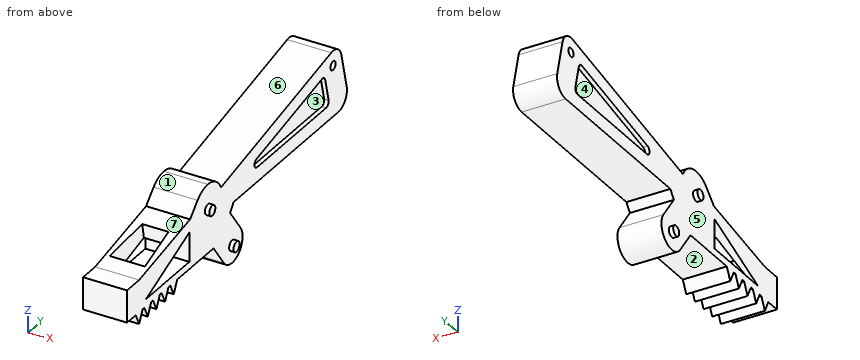
from build123d import *

# Parameters (mm, degrees)
BOSS_EXTRUDE1_DEPTH = 7.5
BOSS_EXTRUDE2_DEPTH = 15
LPATTERN1_COUNT     = 5
LPATTERN1_PITCH     = 5
CUT_EXTRUDE1_DEPTH  = 132.304814948
FILLET1_R           = 8.5
FILLET2_R           = 5
SKETCH4_R           = 1.5
CUT_EXTRUDE2_DEPTH  = 130.82329799
CUT_EXTRUDE3_REACH  = 131.114
SKETCH6_R           = 1.75
BOSS_EXTRUDE3_DEPTH = 1.5
SKETCH7_R           = 1.75
BOSS_EXTRUDE4_DEPTH = 1.5
CUT_EXTRUDE4_DEPTH  = 1.5


with BuildPart() as part:
    # Sketch1 → Boss-Extrude1 (new, symmetric)
    with BuildSketch(Plane(origin=(0, 0, 0), x_dir=(0, 0, -1), z_dir=(1, 0, 0))):
        with BuildLine():
            Line((1.125844004, 128.547240234), (-22.171185278, 122.781095368))
            Line((-22.171185278, 122.781095368), (-7.570249068, 54.320795472))
            Line((-7.570249068, 54.320795472), (-12.460270489, 53.277871457))
            Line((-12.460270489, 53.277871457), (-12.460270489, 43.277871457))
            Line((-12.460270489, 43.277871457), (-5.749067667, 36.443984461))
            Line((-5.749067667, 36.443984461), (0, 7))
            Line((0, 7), (0, 0))
            Line((0, 0), (11, 0))
            Line((11, 0), (11, 50))
            Line((11, 50), (19.022755483, 55.969538882))
            ThreePointArc((19.022755483, 55.969538882), (20.254685443, 64.364915501), (11.859308824, 65.596845461))
            Line((11.859308824, 65.596845461), (3.836553342, 59.627306579))
            Line((3.836553342, 59.627306579), (1.125844004, 61.629450689))
            Line((1.125844004, 61.629450689), (1.125844004, 128.547240234))
        make_face()
    extrude(amount=BOSS_EXTRUDE1_DEPTH, both=True)

    # Sketch2 → Boss-Extrude2 (add)
    with BuildSketch(Plane(origin=(7.5, 0, 0), x_dir=(0, 0, -1), z_dir=(1, 0, 0))):
        Polygon((11, 5), (15, 7), (11, 9), align=None)
    boss_extrude2 = extrude(amount=-BOSS_EXTRUDE2_DEPTH)

    # LPattern1: Boss-Extrude2 ×5
    with Locations(*[(0, i * LPATTERN1_PITCH, 0) for i in range(1, LPATTERN1_COUNT)]):
        add(boss_extrude2)

    # Sketch3 → Cut-Extrude1 (cut, through all)
    with BuildSketch(Plane(origin=(7.5, 0, 0), x_dir=(0, 0, -1), z_dir=(1, 0, 0))):
        Polygon((8.514249155, 11.015619925), (8.514249155, 36.015619925), (-1.485750845, 36.015619925), align=None)
    extrude(amount=-CUT_EXTRUDE1_DEPTH, mode=Mode.SUBTRACT)

    # Fillet1
    # the kernel refuses this fillet: 8.5 mm, written as the material it takes off along each edge
    with BuildSketch(Plane(origin=(-16.189504631, 43.277871457, 12.460270489), x_dir=(0, 1, 0), z_dir=(1, 0, 0))) as fillet1_piece_1:
        with BuildLine():
            CenterArc((FILLET1_R * 0.408917864968, -FILLET1_R), FILLET1_R, 90, 44.481059687)
            Line((-FILLET1_R * 0.29175558125, -FILLET1_R * 0.286517889667), (-FILLET1_R * 0.305769050174, -FILLET1_R * 0.27224824746))
            Line((-FILLET1_R * 0.305769050174, -FILLET1_R * 0.27224824746), (-FILLET1_R * 0.00817835729936, FILLET1_R * 0.02))
            Line((-FILLET1_R * 0.00817835729936, FILLET1_R * 0.02), (FILLET1_R * 0.408917864968, FILLET1_R * 0.02))
            Line((FILLET1_R * 0.408917864968, FILLET1_R * 0.02), (FILLET1_R * 0.408917864968, 0))
        make_face()
    extrude(amount=32.379009261, mode=Mode.SUBTRACT)
    with BuildSketch(Plane(origin=(-24.131006979, 53.277871457, 12.460270489), x_dir=(0, 0.20858480299843193, -0.9780042842227765), z_dir=(1, 0, 0))) as fillet1_piece_2:
        with BuildLine():
            CenterArc((6.92544629, -8.279049256), FILLET1_R, 103.092457682, 64.868111345)
            Line((-1.387590126, -6.506078431), (-1.553850854, -6.470619014))
            Line((-1.553850854, -6.470619014), (-0.166260728, 0.035459417))
            Line((-0.166260728, 0.035459417), (0, 0.17))
            ThreePointArc((0, 0.17), (2.5, 0.17), (4.961491074, 0.165580985))
            Line((4.961491074, 0.165580985), (5, 0))
        make_face()
    extrude(amount=48.262013958, mode=Mode.SUBTRACT)

    # Fillet2
    fillet2_edges = [part.edges().sort_by_distance(p)[0] for p in [
        (0, 122.781095368, 22.171185278),
        (0, 128.547240234, -1.125844004),
    ]]
    fillet(fillet2_edges, radius=FILLET2_R)

    # Sketch4 → Cut-Extrude2 (cut, through all)
    with BuildSketch(Plane(origin=(7.5, 0, 0), x_dir=(0, 0, -1), z_dir=(1, 0, 0))):
        with Locations((-16.271597688, 119.090404926)):
            Circle(SKETCH4_R)
    extrude(amount=-CUT_EXTRUDE2_DEPTH, mode=Mode.SUBTRACT)

    # Cut-Extrude3: up to this plane
    cut_extrude3_end = Plane(origin=(-7.5, 36.015619925, 1.485750845), z_dir=(0, -0.3713906763541038, 0.9284766908852593))
    # Sketch5 → Cut-Extrude3 (cut, up to the surface)
    with BuildSketch(Plane(origin=(0, 0.257069393, -1.316586904), x_dir=(1, 0, 0), z_dir=(0, -0.19163558890630344, 0.9814661487104557)), mode=Mode.PRIVATE) as cut_extrude3_sk1:
        Polygon((4.5, 29.370263041), (-4.5, 29.370263041), (-6, 12.858555839), (6, 12.858555839), align=None)
    cut_extrude3_tool1 = split(extrude(cut_extrude3_sk1.sketch, amount=-CUT_EXTRUDE3_REACH, mode=Mode.PRIVATE), bisect_by=cut_extrude3_end, keep=Keep.BOTH, mode=Mode.PRIVATE)
    add(cut_extrude3_tool1.solids().sort_by_distance((0, 20.594298, 2.654347))[0], mode=Mode.SUBTRACT)

    # Sketch6 → Boss-Extrude3 (add)
    with BuildSketch(Plane(origin=(7.5, 0, 0), x_dir=(0, 0, -1), z_dir=(1, 0, 0))):
        with Locations(Location((15.441032154, 60.783192172, 0), (0, 0, 180))):
            Circle(SKETCH6_R)
    boss_extrude3 = extrude(amount=BOSS_EXTRUDE3_DEPTH)

    # Sketch7 → Boss-Extrude4 (add)
    with BuildSketch(Plane(origin=(7.5, 0, 0), x_dir=(0, 0, -1), z_dir=(1, 0, 0))):
        with Locations(Location((-3.960270489, 46.753673309, 0), (0, 0, 180))):
            Circle(SKETCH7_R)
    boss_extrude4 = extrude(amount=BOSS_EXTRUDE4_DEPTH)

    # Sketch8 → Cut-Extrude4 (cut)
    with BuildSketch(Plane(origin=(7.5, 0, 0), x_dir=(0, 0, -1), z_dir=(1, 0, 0))):
        with BuildLine():
            Line((-14.925252721, 112.777715187), (-6.841162422, 74.873348079))
            ThreePointArc((-6.841162422, 74.873348079), (-5.216849988, 73.694496481), (-3.874155996, 75.186225283))
            Line((-3.874155996, 75.186225283), (-3.874155996, 115.091449891))
            ThreePointArc((-3.874155996, 115.091449891), (-4.449649663, 116.272673004), (-5.73454005, 116.547514222))
            Line((-5.73454005, 116.547514222), (-13.818630348, 114.546656721))
            ThreePointArc((-13.818630348, 114.546656721), (-14.729909587, 113.886125212), (-14.925252721, 112.777715187))
        make_face()
    cut_extrude4 = extrude(amount=-CUT_EXTRUDE4_DEPTH, mode=Mode.SUBTRACT)

    # Mirror1: Boss-Extrude3, Boss-Extrude4, Cut-Extrude4 across plane
    add(boss_extrude3.mirror(Plane(origin=(0, 0, 0), x_dir=(0, 0, 1), z_dir=(1, 0, 0))))
    add(boss_extrude4.mirror(Plane(origin=(0, 0, 0), x_dir=(0, 0, 1), z_dir=(1, 0, 0))))
    add(cut_extrude4.mirror(Plane(origin=(0, 0, 0), x_dir=(0, 0, 1), z_dir=(1, 0, 0))), mode=Mode.SUBTRACT)


solid = part.part
The listing builds one solid part. Answer for the finished solid, in the listing's coordinates (mm). Face numbers are marked on the shaded views. A direction names the side the tool comes from. Coordinates: 2 decimals unless noted, no trailing zeros. Write each loop counter-clockwise with the first axis right and the second up, starting at its lowest first coordinate (ties: lowest second). Pieces come first, ordered by that corner, then holes. Notation, with made-up numbers: M 64,-32.5 L 79,-32.5 A7 ccw 79,-21.5 Z; hole C 25.25,60 d2. An arc over 180 degrees is marked long. Put each result on its own line as item: value. Start each with the question number.
1. A cutting plane is placed at A-A on z = -5.5. Write down the section's boundary in (x, y).
2. A cutting plane is placed at D-D on y = 71. Write down the section's boundary in (x, z).
3. For a pull along Y with two mould halves and no side action, classify the marked faces 5, 6 and 7 as pulls with the +Y half, pulls with the -Y half, needs draft (parallel to the pull), parting line crosses it, or undercut.
4. Which of the six approach directions +Z, -Z, +X, -X, +Y, -Y give full straight-line access (tool end or side, diameter ignored) to the marked faces 1, 2, 3 and 4?
5. A cutting plane is placed at B-B on y = 91.5. Write down the section's boundary in (x, z).
6. Flat-ended cylindrical pins translate along their axes: P1, Ø0.5, axis at x = 2, y = 24.5, coming from the -Z side; P2, Ø7.5, axis at x = 1.5, y = 3.5, coming from the +Z side; P3, Ø1.6, axis at x = -6.5, y = 99.5, coming from the +Z side. Find the tip coordinate at first contact, or state that the pin passes through.
7. A cutting plane is placed at C-C on y = 106. Write down the section's boundary in (x, z), then the cut area to 3 significant figures.
8. Consider line 1 (Z direction, x = 5.5, y = 119); line 2 (Y direction, x = 1, z = -14.5); line 3 (X direction, y = 109.5, z = 3). Determine where each line is inside the solid, lowest interval first. Write a range as from..to.
Resolved:
1. outline: M -7.5,0 L 7.5,0 L 7.5,18.55 L 5.61,18.55 L 6,14.18 L -6,14.18 L -5.61,18.55 L -7.5,18.55 Z; M -7.5,36.02 L 7.5,36.02 L 7.5,60.87 L -7.5,60.87 Z
2. outline: M -7.5,-1.13 L 7.5,-1.13 L 7.5,11.13 L -7.5,11.13 Z
3. face 5: needs draft
3. face 6: undercut
3. face 7: pulls with the -Y half
4. face 1: +Z, +X, -X, -Y
4. face 2: -Z, +X, -X
4. face 3: +X
4. face 4: -X
5. outline: M -7.5,-1.13 L 7.5,-1.13 L 7.5,3.87 L 6,3.87 L 6,10.39 L 7.5,10.39 L 7.5,15.5 L -7.5,15.5 L -7.5,10.39 L -6,10.39 L -6,3.87 L -7.5,3.87 Z
6. P1: stops at z = -11
6. P2: stops at z = 0.05
6. P3: stops at z = 17.38
7. outline: M -7.5,-1.13 L 7.5,-1.13 L 7.5,3.87 L 6,3.87 L 6,13.48 L 7.5,13.48 L 7.5,18.59 L -7.5,18.59 L -7.5,13.48 L -6,13.48 L -6,3.87 L -7.5,3.87 Z
7. area: 267 mm2
8. line 1: z = -1.13..14.77, 17.77..21.27
8. line 2: y = 6.75..7.25, 11.75..12.25, 16.75..17.25, 21.75..22.25, 26.75..27.25, 52.6..66.71
8. line 3: x = -7.5..7.5
